from build123d import *

# Parameters (mm, degrees)
CYLINDER020_R             = 3.1
CYLINDER020_DEPTH         = 3
CYLINDER021_R             = 3.1
CYLINDER021_DEPTH         = 3
CYLINDER022_R             = 1.7
CYLINDER022_DEPTH         = 21
BOX003_W                  = 23
BOX003_H                  = 5.2
BOX003_DEPTH              = 3
PRISM_DEPTH               = 3
FUSION006_PLACEMENT_ANGLE = 90
CYLINDER006_R             = 4.05
CYLINDER006_DEPTH         = 270
EXTRUDE_DEPTH             = 60
BOX002_W                  = 43
BOX002_H                  = 12
BOX002_DEPTH              = 16
BOX_W                     = 16
BOX_H                     = 19
BOX_DEPTH                 = 16
FILLET_R                  = 3
FILLET001_R               = 2


with BuildPart() as cilindro020:
    # Cylinder020 → Cylinder020 (new body)
    with BuildSketch(Plane(origin=(35, 6, 62), x_dir=(1, 0, 0), z_dir=(0, 0, -1))):
        Circle(CYLINDER020_R)
    extrude(amount=CYLINDER020_DEPTH)


with BuildPart() as cilindro021:
    # Cylinder021 → Cylinder021 (new body)
    with BuildSketch(Plane(origin=(15, -6, 62), x_dir=(1, 0, 0), z_dir=(0, 0, -1))):
        Circle(CYLINDER021_R)
    extrude(amount=CYLINDER021_DEPTH)


with BuildPart() as cilindro022:
    # Cylinder022 → Cylinder022 (new body)
    with BuildSketch(Plane.XY.offset(-6)):
        Circle(CYLINDER022_R)
    extrude(amount=CYLINDER022_DEPTH)


with BuildPart() as cubo003:
    # Box003 → Box003 (new body)
    with BuildSketch(Plane(origin=(0, -2.6, 0), x_dir=(1, 0, 0), z_dir=(0, 0, 1))):
        with Locations((11.5, 2.6)):
            Rectangle(BOX003_W, BOX003_H)
    extrude(amount=BOX003_DEPTH)


with BuildPart() as hueco_tornillo:
    # Prism → Prism (new body)
    with BuildSketch(Plane.XY):
        Polygon((3, 0), (1.5, 2.598076), (-1.5, 2.598076), (-3, 0), (-1.5, -2.598076), (1.5, -2.598076), align=None)
    extrude(amount=PRISM_DEPTH)

    # Fusion006: union Cilindro022, Cubo003
    add(cilindro022.part)
    add(cubo003.part)


with BuildPart() as hueco_tornillo_1:
    # Fusion006 placement: moved
    add(hueco_tornillo.part.moved(Location((-43, 7, 71))).rotate(Axis((-43, 7, 71), (-1, 0, 0)), FUSION006_PLACEMENT_ANGLE))


with BuildPart() as fusion005:
    # Cylinder006 → Cylinder006 (new body)
    with BuildSketch(Plane(origin=(-51, 0, 71), x_dir=(0, 0, -1), z_dir=(1, 0, 0))):
        Circle(CYLINDER006_R)
    extrude(amount=CYLINDER006_DEPTH)

    # Fusion005: union Cilindro020, Cilindro021, hueco_tornillo
    add(cilindro020.part)
    add(cilindro021.part)
    add(hueco_tornillo_1.part)


with BuildPart() as extrude_body:
    # Sketch → Extrude (new body, symmetric)
    with BuildSketch(Plane.XZ):
        with BuildLine():
            Line((-51, 61), (42, 61))
            Line((42, 61), (42, 55))
            ThreePointArc((-51, 54.267), (-4.382542, 39.730934), (42, 55))
            Line((-51, 61), (-51, 54.267))
        make_face()
    extrude(amount=EXTRUDE_DEPTH, both=True)


with BuildPart() as cubo002:
    # Box002 → Box002 (new body)
    with BuildSketch(Plane(origin=(-35, -6, 61), x_dir=(1, 0, 0), z_dir=(0, 0, 1))):
        with Locations((21.5, 6)):
            Rectangle(BOX002_W, BOX002_H)
    extrude(amount=BOX002_DEPTH)


with BuildPart() as fillet001:
    # Box → Box (new body)
    with BuildSketch(Plane(origin=(-51, -6, 61), x_dir=(1, 0, 0), z_dir=(0, 0, 1))):
        with Locations((8, 9.5)):
            Rectangle(BOX_W, BOX_H)
    extrude(amount=BOX_DEPTH)

    # Fusion002: union Extrude body, Cubo002
    add(extrude_body.part)
    add(cubo002.part)

    # Cut006: cut Fusion005
    add(fusion005.part, mode=Mode.SUBTRACT)

    # Fillet
    fillet_edges = [fillet001.edges().sort_by_distance(p)[0] for p in [
        (-4.5, 60, 61),
        (42, 0, 61),
        (-4.5, -60, 61),
        (42, 60, 58),
        (-4.382542, 60, 39.730934),
        (42, 0, 55),
        (42, -60, 58),
        (-4.382542, -60, 39.730934),
    ]]
    fillet(fillet_edges, radius=FILLET_R)

    # Fillet001
    fillet001_edges = [fillet001.edges().sort_by_distance(p)[0] for p in [
        (-43, 13, 61),
        (-35, 9.5, 61),
        (-13.5, 6, 61),
        (-21.5, -6, 61),
        (-35, 13, 69),
        (-43, 13, 77),
        (-35, 9.5, 77),
        (-13.5, 6, 77),
        (-21.5, -6, 77),
    ]]
    fillet(fillet001_edges, radius=FILLET001_R)


solid = fillet001.part
Work out the finished part from the listing and answer in its coordinate system (mm). A direction names the side the tool comes from. Round coordinates to 2 decimals unless told otherwise and drop trailing zeros. Write each loop counter-clockwise with the first axis right and the second up, starting at its lowest first coordinate (ties: lowest second). Pieces come first, ordered by that corner, then holes. Notation, with made-up numbers: (35, -7) -> (47, -7) arc R17 cw to (47, -3) -> close; hole circle Ø10 at (78.25, -25.5). An arc over 180 degrees is marked (long way). Answer as CSV lines item,"result". Start each with the question number.
(1) The mould has two halves that part along X. Classify faces 1 (the flat face through (8, -2, 67)), 2 (the flat face through (-22, -6, 69)), 3 (the cylindrical face through (32.54, 7.886, 60.014)): +X half, -X half, draft (parallel to the pull), parting line (faces both ways), or undercut.
(2) A tool of negligible diameter and unlimited length cuts with its end or side. For faces 4 (the flat face through (-14, 6, 69)), 5 (the flat face through (-45.24, 8.48, 69.68)), 6 (the cylindrical face through (-44.25, 11.48, 69.85)), 7 (the cylindrical face through (-5.37, 59.1, 60.14)), 8 (the cylindrical face through (14.328, -2.974, 60.014)), from which of +Z, -Z, +X, -X, +Y, -Y can it reach the whole face along a straight path? Write none if from no direction.
(3) Find the intervals of material crossed by probe 1 along X at (y, z) = (5, 71); probe 2 along Y at (x, z) = (-32.5, 71); probe 3 along Y at (x, z) = (-7.5, 74.5), in increasing order.
(4) Each of these flat-tipped pins is pushed along its axis until it touches: pin 1 (5.5 mm diameter, centred on x = -42, z = 72, fed in from +Y); pin 2 (1.9 mm diameter, centred on x = 14, y = -5, fed in from +Z); pin 3 (4 mm diameter, centred on y = 7.5, z = 66.5, fed in from +X). Where does it stop, or does it pass through?
(5) The part is cut by section A-A, the plane z = 65. Give the vertices of the cut face in (x, y).
(6) The part is cut by section B-B, the plane y = -21. Give the vertices of the cut face in (x, z), then the cut area to 3 significant figures.
Output values:
1,face 1,"+X half"
1,face 2,"draft"
1,face 3,"undercut"
2,face 4,"+Z, +X, +Y"
2,face 5,"+X"
2,face 6,"+Y"
2,face 7,"+Z, +X, -X, +Y"
2,face 8,"+Z"
3,probe 1,"x = -51 to -44.7, -41.3 to 8"
3,probe 2,"y = -6 to -4.05, 4.05 to 6"
3,probe 3,"y = -6 to -2.04, 2.04 to 6"
4,pin 1,"stops at y = 13"
4,pin 2,"stops at z = 59"
4,pin 3,"stops at x = 8"
5,outline,"(-51, -6) -> (8, -6) -> (8, 6) -> (-35, 6) -> (-35, 11) arc R2 ccw to (-37, 13) -> (-51, 13) -> close"
6,outline,"(-51, 54.27) arc R80 ccw to (40.71, 54.09) arc R3 ccw to (42, 56.55) -> (42, 58) arc R3 ccw to (39, 61) -> (-51, 61) -> close"
6,area,"1,530 mm²"
